```python
from build123d import *

# Parameters (mm, degrees)
BOSS_EXTRUDE1_DEPTH = 107.95
SKETCH2_W           = 31.75
SKETCH2_H           = 15.875
CUT_EXTRUDE1_DEPTH  = 127
SKETCH3_OUTSIDE_W   = 91.34
SKETCH3_OUTSIDE_H   = 59.59
SKETCH3_OUTSIDE_R   = 28.575
CUT_EXTRUDE2_DEPTH  = 108.95


with BuildPart() as part:
    # Sketch1 → Boss-Extrude1 (new body)
    with BuildSketch(Plane(origin=(0, 0, 0), x_dir=(0, 0, -1), z_dir=(1, 0, 0))):
        with BuildLine():
            Line((-25.4, 0), (-31.75, 0))
            ThreePointArc((-31.75, 0), (0, -31.75), (31.75, 0))
            Line((31.75, 0), (25.4, 0))
            ThreePointArc((25.4, 0), (0, -25.4), (-25.4, 0))
        make_face()
    extrude(amount=-BOSS_EXTRUDE1_DEPTH)

    # Sketch2 → Cut-Extrude1 (cut)
    with BuildSketch(Plane.XY):
        with Locations((-15.875, -7.9375)):
            Rectangle(SKETCH2_W, SKETCH2_H)
    extrude(amount=CUT_EXTRUDE1_DEPTH, mode=Mode.SUBTRACT)

    # Sketch3 outside → Cut-Extrude2 (cut, through all)
    with BuildSketch(Plane(origin=(0, 0, 0), x_dir=(0, 0, -1), z_dir=(1, 0, 0))):
        with Locations((0, -15.875)):
            Rectangle(SKETCH3_OUTSIDE_W, SKETCH3_OUTSIDE_H)
        Circle(SKETCH3_OUTSIDE_R, mode=Mode.SUBTRACT)
    extrude(amount=-CUT_EXTRUDE2_DEPTH, mode=Mode.SUBTRACT)


solid = part.part
```
Verification items for the finished model (mm, model axes). A direction names the side the tool comes from. Give positions to 0.01 mm unless a question says otherwise; leave off trailing zeros. Write each loop counter-clockwise with the first axis right and the second up, starting at its lowest first coordinate (ties: lowest second). Pieces come first, ordered by that corner, then holes. Notation, with made-up numbers: M 10.5,-27 L 45.5,-27 A25 cw 45.5,5 Z; hole C -6,37.5 d2. An arc over 180 degrees is marked long. One line per question, with ' | ' between items.
1) Section check A-A on y = -6.75. Enter the section's corners in (x, z), plus the area to 3 significant figures.
Result:
outline: M -107.95,-27.77 L 0,-27.77 L 0,-24.49 L -107.95,-24.49 Z; M -107.95,24.49 L -31.75,24.49 L -31.75,27.77 L -107.95,27.77 Z | area: 604 mm2
2) Section check C-C on x = -49.5. Enter the section's corners in (y, z) (3 decimals), plus the area to 3 significant figures.
Result:
outline: M 0,-28.575 L 0,-25.4 A25.4 cw 0,25.4 L 0,28.575 A28.575 ccw Z | area: 269 mm2
3) Thickness scan on line 1 along Z through (x, y) = (-82, -22); line 2 along Z through (x, y) = (-79, -8); line 3 along Y through (x, z) = (-36.5, -0.5). Record the ranges inside material, lowest first. Write a range as [from, to].
Result:
line 1: z = [-18.24, -12.69], [12.69, 18.24] | line 2: z = [-27.43, -24.11], [24.11, 27.43] | line 3: y = [-28.57, -25.4]
4) Set-up check for faces 4 (the flat face through (-31.75, -8, 25)), 5 (the flat face through (0, -24, -10)): record each of +Z, -Z, +X, -X, +Y, -Y from which the full face is reachable in a straight line by a thin tool's end or side.
Result:
face 4: +Z, +X, +Y | face 5: +Z, -Z, +X, +Y, -Y
5) Gauge pin test, flat ends, axial feed: pin 1 Ø4 at (x, z) = (-40, -1.5) entering from +Y; pin 2 Ø3 at (x, y) = (-41, -7.5) entering from -Z; pin 3 Ø9.5 at (y, z) = (-10, 23.5) entering from +X. Record the tip position at first contact, or that the pin passes through.
Result:
pin 1: stops at y = -25.16 | pin 2: stops at z = -27.94 | pin 3: stops at x = -31.75
6) Mould release check, pull along Z, two halves, no side actions. Record for faces 1 (the cylindrical face through (-53.219, -25.394, -0.559)), 2 (the cylindrical face through (-53.22, -28.57, -0.63)), 3 (the flat face through (-69, 0, 27)): released by +Z, released by -Z, zero draft, split by the parting line, or undercut.
Result:
face 1: undercut | face 2: split by the parting line | face 3: zero draft
7) Section check B-B on z = 0. Enter the section's corners in (x, y) (3 decimals).
Result:
outline: M -107.95,-28.575 L 0,-28.575 L 0,-25.4 L -107.95,-25.4 Z
